Could you check a few things on this model? Use its own coordinates, in mm. Face numbers are marked on the shaded views. Round coordinates to 2 decimals unless told otherwise and drop trailing zeros. Order: outer loops, then holes, each group sorted by start corner. A loop starts at its lowest first (then second) coordinate and runs counter-clockwise, first axis right, second up. Notation, with made-up numbers: M -6,46 L 3,46 A18 cw 3,50 Z; hole C 87,53 d3. An arc over 180 degrees is marked long. Write each question's results on one line, items separated by ' | '. Start each with the question number.
1. I'm going to push flat-ended pins straight in: pin 1 (5 mm diameter, centred on x = 9, y = -18, fed in from -Z); pin 2 (4 mm diameter, centred on y = -25.5, z = 17, fed in from +X); pin 3 (3 mm diameter, centred on y = 3.5, z = 10, fed in from +X); pin 4 (3 mm diameter, centred on x = -18, y = -17, fed in from +Z). Where does each tip first touch, or does it pass through?
2. Suppose I cut it at A-A on y = 0. Write out the boundary of the cut face in (x, z), and give its area (3 significant figures).
3. We'd pull the mould along Y, two halves only. Please class the marked faces 1, 2 and 3: released by +Y, released by -Y, zero draft, split by the parting line, or undercut.
4. Suppose I cut it at D-D on z = 14.2. Write out the boundary of the cut face in (x, y), and give its area (3 significant figures).
5. Suppose I cut it at C-C on z = 30. Write out the boundary of the cut face in (x, y).
6. Please list where these lines run through material, in increasing order: L1, parallel to X at y = 19.5, z = 41.5; L2, parallel to Z at x = 14, y = 0; L3, parallel to Y at x = -25, z = 41.
7. Suppose I cut it at B-B on x = 0. Write out the boundary of the cut face in (y, z).
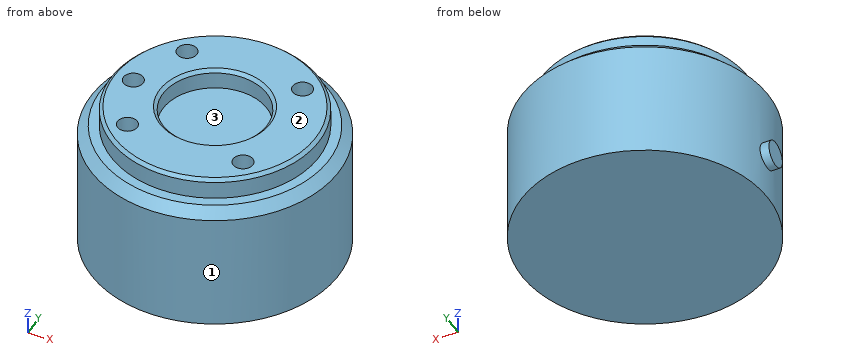
Autodesk Inventor part; units mm, degrees
ref_plane "YZ Plane" through (0, 0, 0) normal (1, 0, 0) x (0, 1, 0)
ref_plane "XZ Plane" through (0, 0, 0) normal (0, 1, 0) x (-1, 0, 0)
ref_plane "XY Plane" through (0, 0, 0) normal (0, 0, 1) x (1, 0, 0)
sketch "スケッチ1" plane through (0, 0, 0) normal (0, 0, 1) x (1, 0, 0)
  circle A0 centre (0, 0) radius 37.5
  dimension "d0" = 75
extrude "押し出し1" add sketch "スケッチ1" along normal blind 45.75
sketch "スケッチ2" plane through (0, 0, 45.75) normal (0, 0, 1) x (1, 0, 0)
  circle A0 centre (0, 0) radius 37.5
  circle A1 centre (0, 0) radius 31.5
  dimension "d3" = 63
extrude "押し出し2" cut sketch "スケッチ2" against normal blind 6.5
chamfer "面取り1" distance 3 angle 45 1 edges at (-37.5, 0, 39.25)
chamfer "面取り2" distance 1 angle 45 1 edges at (-31.5, 0, 45.75)
sketch "スケッチ3" plane through (0, 0, 45.75) normal (0, 0, 1) x (1, 0, 0)
  circle A0 centre (0, 0) radius 15.75
  dimension "d12" = 31.5
extrude "押し出し3" cut sketch "スケッチ3" against normal blind 6.2
chamfer "面取り3" distance 1 angle 45 1 edges at (-15.75, 0, 45.75)
sketch "スケッチ4" plane through (0, 0, 45.75) normal (0, 0, 1) x (1, 0, 0)
  circle A0 centre (-25, 0) radius 3
  point P0 (0, 0)
  dimension "d18" = 6
extrude "押し出し4" cut sketch "スケッチ4" against normal blind 6.2
sketch "スケッチ5" plane through (0, 0, 45.75) normal (0, 0, 1) x (1, 0, 0)
  point P0 (0, 0)
sketch "スケッチ6" plane through (0, 0, 45.75) normal (0, 0, 1) x (1, 0, 0)
  circle A0 centre (0, 0) radius 25
  circle A1 centre (0, 0) radius 37.5
  line L0 (0, 0) -> (-17.6777, 17.6777)
  line L1 (0, 0) -> (25, 0) construction
  circle A2 centre (-17.6777, 17.6777) radius 3
  circle A3 centre (17.6777, 17.6777) radius 3
  circle A4 centre (17.6777, -17.6777) radius 3
  circle A5 centre (-17.6777, -17.6777) radius 3
  dimension "d21" = 50
  dimension "d22" = 135
  dimension "d23" = 6
  dimension "d24" = 6
  dimension "d25" = 6
  dimension "d26" = 6
extrude "押し出し5" cut sketch "スケッチ6" against normal blind 8 contours A3 A0 | A0 A3 | A4 A0 | A0 A4 | A2 L0 A0 | A0 A2 | A5 A0 | A0 A5 | L0 A2 A0
thread "ねじ1"
thread "ねじ2"
thread "ねじ3"
thread "ねじ4"
sketch "スケッチ7" plane through (0, 0, 0) normal (1, 0, 0) x (0, 1, 0)
  circle A0 centre (0, 14.2) radius 4
  point P0 (0, 0)
  dimension "d37" = 8
extrude "押し出し6" add sketch "スケッチ7" against normal blind 40
properties part number "tool-output-flange"
Filled sheet:
1) pin 1: stops at z = 0 | pin 2: stops at x = 29.22 | pin 3: stops at x = 37.45 | pin 4: stops at z = 37.75
2) outline: M -40,10.2 L -37.5,10.2 L -37.5,0 L 37.5,0 L 37.5,36.25 L 34.5,39.25 L 31.5,39.25 L 31.5,44.75 L 30.5,45.75 L 16.75,45.75 L 15.75,44.75 L 15.75,39.55 L -15.75,39.55 L -15.75,44.75 L -16.75,45.75 L -22,45.75 L -22,39.55 L -28,39.55 L -28,45.75 L -30.5,45.75 L -31.5,44.75 L -31.5,39.25 L -34.5,39.25 L -37.5,36.25 L -37.5,18.2 L -40,18.2 Z | area: 3,130 mm^2
3) face 1: split by the parting line | face 2: zero draft | face 3: undercut
4) outline: M -40,-4 L -37.29,-4 A37.5 ccw long -37.29,4 L -40,4 Z | area: 4,440 mm^2
5) outline: C 0,0 d75
6) L1: x = -24.74 to -20.06, -15.29 to 15.29, 20.06 to 24.74 | L2: z = 0 to 39.55 | L3: y = -19.16 to -3, 3 to 19.16
7) outline: M -37.5,0 L 37.5,0 L 37.5,36.25 L 34.5,39.25 L 31.5,39.25 L 31.5,44.75 L 30.5,45.75 L 16.75,45.75 L 15.75,44.75 L 15.75,39.55 L -15.75,39.55 L -15.75,44.75 L -16.75,45.75 L -30.5,45.75 L -31.5,44.75 L -31.5,39.25 L -34.5,39.25 L -37.5,36.25 Z
